The listing builds one solid part. Answer for the finished solid, in the listing's coordinates (mm). A direction names the side the tool comes from. Round coordinates to 2 decimals unless told otherwise and drop trailing zeros. Loops run counter-clockwise (first coordinate to the right, second up) from the corner with the lowest first, then second, coordinate; pieces in that order, holes last. Notation, with made-up numbers: (4.25, 71) - (18.25, 71) arc R27 cw to (18.25, 89) - close; hole circle Ø10 at (-10.5, 3.5). An arc over 180 degrees is marked (long way). One line per item, written item: value.
Autodesk Inventor part; units mm, degrees
ref_plane "YZ Plane" through (0, 0, 0) normal (1, 0, 0) x (0, 1, 0)
ref_plane "XZ Plane" through (0, 0, 0) normal (0, 1, 0) x (-1, 0, 0)
ref_plane "XY Plane" through (0, 0, 0) normal (0, 0, 1) x (1, 0, 0)
sketch "スケッチ1" plane through (0, 0, 0) normal (0, 1, 0) x (-1, 0, 0)
  circle A0 centre (0, 0) radius 38
  circle A1 centre (0, 0) radius 41
  dimension "d0" = 76
  dimension "d1" = 82
extrude "押し出し1" add sketch "スケッチ1" along normal blind 10
sketch "スケッチ2" plane through (0, 10, 0) normal (0, 1, 0) x (1, 0, 0)
  circle A0 centre (0, 0) radius 41
extrude "押し出し2" add sketch "スケッチ2" along normal blind 2
sketch "スケッチ3" plane through (0, 12, 0) normal (0, 1, 0) x (1, 0, 0)
  circle A0 centre (0, 0) radius 41
sketch "スケッチ4" plane through (0, 12, 0) normal (0, 1, 0) x (1, 0, 0)
  circle A0 centre (0, 0) radius 41
  circle A1 centre (0, 0) radius 20
  dimension "d6" = 40
extrude "押し出し3" cut sketch "スケッチ4" against normal blind 10 contours A1
sketch "スケッチ5" plane through (0, 12, 0) normal (0, 1, 0) x (1, 0, 0)
  circle A0 centre (0, 0) radius 20
  circle A1 centre (0, 0) radius 41
  circle A2 centre (0, 0) radius 30
  dimension "d9" = 60
extrude "押し出し4" add sketch "スケッチ5" along normal blind 1 contours A2
properties part number "知能ロボコン大砲３"
1) For a pull along X with two mould halves and no side action, classify faces 1 (the flat face through (6, 13, 20)), 2 (the flat face through (16, 10, 16)), 3 (the cylindrical face through (-29.97, 12.49, 1.32)) as released by +X, released by -X, zero draft, split by the parting line, or undercut.
Final values:
face 1: zero draft
face 2: undercut
face 3: split by the parting line
2) Consider L1, parallel to Z at x = 0, y = 6; L2, parallel to Z at x = 0, y = 11.45; L3, parallel to X at y = 12.2, z = 0. Determine where each line is inside the solid, lowest interval first.
Final values:
L1: -41 to -38, 38 to 41
L2: -41 to -20, 20 to 41
L3: -30 to -20, 20 to 30
3) Each of these flat-tipped pins is pushed along its axis until it touches: pin 1 Ø2 at (x, z) = (-29, -13) entering from +Y; pin 2 Ø3 at (x, y) = (-27, 8) entering from -Z; pin 3 Ø2 at (y, z) = (6, -1) entering from +X; pin 4 Ø6 at (x, z) = (12.5, 31) entering from -Y. Where does it stop, or does it pass through?
Final values:
pin 1: y = 12
pin 2: z = -32.11
pin 3: x = 41
pin 4: y = 10
4) A cutting plane is placed at C-C on z = -25.5. Give the vertices of the cut face in (x, y), and give its area (3 significant figures).
Final values:
outline: (-32.11, 0) - (-28.17, 0) - (-28.17, 10) - (28.17, 10) - (28.17, 0) - (32.11, 0) - (32.11, 12) - (15.8, 12) - (15.8, 13) - (-15.8, 13) - (-15.8, 12) - (-32.11, 12) - close
area: 239 mm2
5) For faces 4 (the flat face through (2.8, 12, 30.2)), 5 (the cylindrical face through (-17.535, 4.93, 33.713)), 6 (the flat face through (-12, 0, -36.3)), determine the directions among +Z, -Z, +X, -X, +Y, -Y from which every point of the face is accessible in a straight line to the end or side of a thin tool.
Final values:
face 4: +Y
face 5: -Y
face 6: +Z, -Z, +X, -X, -Y
6) A cutting plane is placed at A-A on y = 3.75. Give the vertices of the cut face in (x, z).
Final values:
outline: circle Ø82 at (0, 0); hole circle Ø76 at (0, 0)
